Source: CAD feature listing. Evaluate the final solid. Frame: model axes, mm. A direction names the side the tool comes from. Give positions to 0.01 mm unless a question says otherwise; leave off trailing zeros. Order: outer loops, then holes, each group sorted by start corner. A loop starts at its lowest first (then second) coordinate and runs counter-clockwise, first axis right, second up.
Autodesk Inventor part; units mm, degrees
ref_plane "YZ Plane" through (0, 0, 0) normal (1, 0, 0) x (0, 1, 0)
ref_plane "XZ Plane" through (0, 0, 0) normal (0, 1, 0) x (-1, 0, 0)
ref_plane "XY Plane" through (0, 0, 0) normal (0, 0, 1) x (1, 0, 0)
sketch "Sketch1" plane through (0, 0, 0) normal (0, 0, 1) x (1, 0, 0)
  line L0 (0, 0) -> (38.1, 0)
  line L1 (38.1, 0) -> (38.1, 19.05)
  line L2 (38.1, 19.05) -> (0, 19.05)
  line L3 (0, 19.05) -> (0, 0)
  line L4 (3.175, 15.875) -> (34.925, 15.875)
  line L5 (34.925, 15.875) -> (34.925, 3.175)
  line L6 (34.925, 3.175) -> (3.175, 3.175)
  line L7 (3.175, 3.175) -> (3.175, 15.875)
  dimension "d0" = 38.1
  dimension "d1" = 19.05
  dimension "d2" = 3.175
extrude "Extrusion1" add sketch "Sketch1" along normal blind 381
sketch "Sketch2" plane through (38.1, 0, 0) normal (1, 0, 0) x (0, 0, -1)
  circle A0 centre (-190.5, 9.525) radius 5
  line L0 (0, 19.05) -> (-381, 19.05)
  line L1 (-381, 0) -> (-381, 19.05)
  point P0 (0, 0)
  point P1 (-381, 9.525)
  dimension "d5" = 10
  dimension "d6" = 9.525
  dimension "d7" = 190.5
extrude "Extrusion2" cut sketch "Sketch2" against normal blind 381
sketch "Sketch4" plane through (38.1, 0, 0) normal (1, 0, 0) x (0, 0, -1)
  line L0 (-381, 0) -> (-381, 19.05)
  line L1 (-381, 9.525) -> (-254, 9.525)
  circle A0 centre (-368.3, 9.525) radius 2.5
  circle A1 centre (-332.74, 9.525) radius 2.5
  circle A2 centre (-297.18, 9.525) radius 2.5
  circle A3 centre (-261.62, 9.525) radius 2.5
  circle A4 centre (-226.06, 9.525) radius 2.5
  line L2 (0, 0) -> (0, 19.05)
  line L3 (0, 9.525) -> (-40.9904, 9.525)
  circle A5 centre (-12.7, 9.525) radius 2.5
  circle A6 centre (-48.26, 9.525) radius 2.5
  circle A7 centre (-83.82, 9.525) radius 2.5
  circle A8 centre (-119.38, 9.525) radius 2.5
  circle A9 centre (-154.94, 9.525) radius 2.5
  dimension "d10" = 127
  dimension "d11" = 5
  dimension "d14" = 35.56
  dimension "d19" = 12.7
  dimension "d20" = 5
  dimension "d23" = 35.56
  dimension "d28" = 12.7
extrude "Extrusion3" cut sketch "Sketch4" against normal blind 381
properties part number "hinge aray side"
1) Reachability of faces 4 (the face through (0, 16, 188)), 5 (the face through (3.175, 5, 188)) from +Z, -Z, +X, -X, +Y, -Y: full face, straight path, thin tool, end or side. Return the list, or none.
Checks:
face 4: +Z, -Z, -X, +Y, -Y
face 5: +Z, -Z
2) Ray query, L1, parallel to Y at x = 18, z = 93 (3 decimals); L2, parallel to X at y = 7.75, z = 92.5 (3 decimals); L3, parallel to Y at x = 37.1, z = 83.82 (3 decimals). Return the intervals inside material, ascending.
Checks:
L1: y = 0 to 3.175, 15.875 to 19.05
L2: x = 0 to 3.175, 34.925 to 38.1
L3: y = 0 to 7.025, 12.025 to 19.05
3) Section query C-C on z = 70. Output: boundary loops of the cut face in (x, y) (3 decimals).
Checks:
outline: (0, 0) - (38.1, 0) - (38.1, 19.05) - (0, 19.05) - close; hole (3.175, 3.175) - (34.925, 3.175) - (34.925, 15.875) - (3.175, 15.875) - close
4) Pull-direction query (X, two-part tool) for faces 1 (the face through (19, 18, 381)), 2 (the face through (38.1, 5, 188)), 3 (the face through (34.925, 15, 188)); classes: +X half, -X half, draft (parallel to the pull), parting line (faces both ways), or undercut.
Checks:
face 1: draft
face 2: +X half
face 3: undercut
5) Section query A-A on z = 190.5. Output: boundary loops of the cut face in (x, y) (3 decimals).
Checks:
outline: (0, 0) - (38.1, 0) - (38.1, 4.525) - (34.925, 4.525) - (34.925, 3.175) - (3.175, 3.175) - (3.175, 4.525) - (0, 4.525) - close; (0, 14.525) - (3.175, 14.525) - (3.175, 15.875) - (34.925, 15.875) - (34.925, 14.525) - (38.1, 14.525) - (38.1, 19.05) - (0, 19.05) - close
6) Section query B-B on x = 17. Output: boundary loops of the cut face in (y, z) (3 decimals), and give its area (3 significant figures).
Checks:
outline: (0, 0) - (3.175, 0) - (3.175, 381) - (0, 381) - close; (15.875, 0) - (19.05, 0) - (19.05, 381) - (15.875, 381) - close
area: 2,420 mm2
